Can you work these out from the model? Positions are in its coordinate system, mm. Round coordinates to 2 decimals unless told otherwise and drop trailing zeros. Write each loop counter-clockwise with the first axis right and the second up, starting at its lowest first coordinate (ties: lowest second). Pieces come first, ordered by that corner, then holes. Notation, with made-up numbers: (50, 22.25) -> (109, 22.25) arc R13 cw to (109, 37.25) -> close; hole circle Ø2 at (-7, 42). An arc over 180 degrees is marked (long way). Write item = value, one per line. Start each with the question number.
1) I'm going to push a flat-ended pin straight in: pin 1 (12 mm diameter, centred on x = 12, y = -1.5, fed in from -Z). Where does the tip first touch, or does it pass through?
2) Imagine slicing it at B-B, the plane x = 0. Please give me the cut outline in (y, z), then the cut area to 3 significant figures.
3) Imagine slicing it at A-A, the plane y = -36.5. Please give me the cut outline in (x, z).
4) If I drill on line 1 (Y direction, x = 0, z = 0.55); line 2 (X direction, y = 36.5, z = 0.45); line 3 (X direction, y = -35.5, z = 0.85), over which ranges is the centre line in solid material (lowest first)?
Autodesk Inventor part; units mm, degrees
ref_plane "YZ Plane" through (0, 0, 0) normal (1, 0, 0) x (0, 1, 0)
ref_plane "XZ Plane" through (0, 0, 0) normal (0, 1, 0) x (-1, 0, 0)
ref_plane "XY Plane" through (0, 0, 0) normal (0, 0, 1) x (1, 0, 0)
sketch "스케치1" plane through (0, 0, 0) normal (0, 0, 1) x (1, 0, 0)
  point P0 (0, 0)
sketch "스케치2" plane through (0, 0, 0) normal (0, 0, 1) x (1, 0, 0)
  line L0 (-26, 44.5) -> (26, 44.5)
  line L1 (26, 44.5) -> (26, -44.5)
  line L2 (26, -44.5) -> (-26, -44.5)
  line L3 (-26, -44.5) -> (-26, 44.5)
  line L4 (-26, 44.5) -> (26, -44.5) construction
  line L5 (26, 44.5) -> (-26, -44.5) construction
  point P0 (0, 0)
  dimension "d0" = 52
  dimension "d1" = 89
extrude "돌출1" add sketch "스케치2" along normal blind 1.6
sketch "스케치3" plane through (0, 0, 1.6) normal (0, 0, 1) x (1, 0, 0)
  circle A0 centre (0, 36.5) radius 1.5
  line L0 (26, 44.5) -> (-26, 44.5)
  circle A1 centre (0, -36.5) radius 1.5
  line L1 (-26, -44.5) -> (26, -44.5)
  line L2 (0, -62.3) -> (0, 62.3)
  point P0 (0, 0)
  dimension "d4" = 3
  dimension "d5" = 8
  dimension "d6" = 3
  dimension "d7" = 8
extrude "돌출2" cut sketch "스케치3" against normal up to surface (1.6 mm away)
properties part number "빵판"
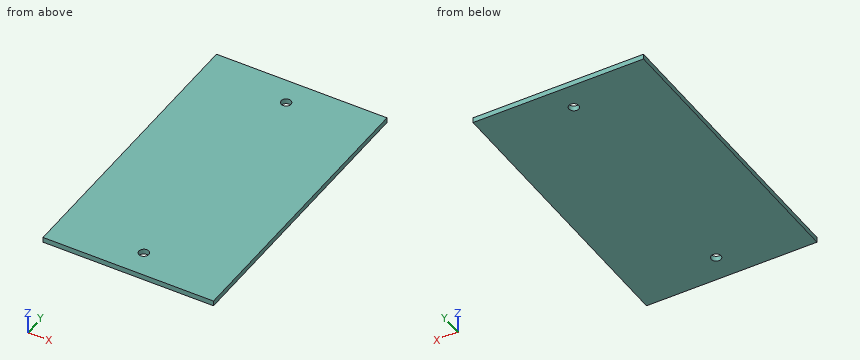
Reported:
q1.pin_1 = 0
q2.outline = (-44.5, 0) -> (-38, 0) -> (-38, 1.6) -> (-44.5, 1.6) -> close; (-35, 0) -> (35, 0) -> (35, 1.6) -> (-35, 1.6) -> close; (38, 0) -> (44.5, 0) -> (44.5, 1.6) -> (38, 1.6) -> close
q2.area = 133 mm²
q3.outline = (-26, 0) -> (-1.5, 0) -> (-1.5, 1.6) -> (-26, 1.6) -> close; (1.5, 0) -> (26, 0) -> (26, 1.6) -> (1.5, 1.6) -> close
q4.line_1 = -44.5 to -38, -35 to 35, 38 to 44.5
q4.line_2 = -26 to -1.5, 1.5 to 26
q4.line_3 = -26 to -1.12, 1.12 to 26
